from build123d import *

# Parameters (mm, degrees)
F1_DEPTH = 30
F3_DEPTH = 4.4
F4_DEPTH = 2
F5_DEPTH = 2.4
F7_DEPTH = 4.4


with BuildPart() as f1:
    # F0 (on Top) → F1 (new body)
    with BuildSketch(Plane.XY):
        with BuildLine():
            Line((7.8582108495, 2.1976148234), (7.8582108495, 1.5812813318))
            Line((7.8582108495, 1.5812813318), (7.8582108495, -2.1976148234))
            ThreePointArc((7.8582108495, -2.1976148234), (12.3474105352, -3.8320303136), (15.2004390117, 0))
            ThreePointArc((15.2004390117, 0), (12.3474105352, 3.8320303136), (7.8582108495, 2.1976148234))
        make_face()
        with BuildLine():
            ThreePointArc((8.9505391584, 1.5812813318), (12.0296782424, 2.6219958616), (13.9504390117, 0))
            ThreePointArc((13.9504390117, 0), (10.3711997809, -2.6219958616), (8.9505391584, 1.5812813318))
        make_face(mode=Mode.SUBTRACT)
        with BuildLine():
            Line((7.8582108495, -2.1976148234), (7.8582108495, 1.5812813318))
            Line((7.8582108495, 1.5812813318), (7.5262657237, 1.5812813318))
            ThreePointArc((7.5262657237, 1.5812813318), (7.2157826444, -0.3500194778), (7.8582108495, -2.1976148234))
        make_face()
        with BuildLine():
            Line((7.5262657237, 1.5812813318), (7.8582108495, 1.5812813318))
            Line((7.8582108495, 1.5812813318), (7.8582108495, 2.1976148234))
            ThreePointArc((7.8582108495, 2.1976148234), (7.6787293316, 1.8967237357), (7.5262657237, 1.5812813318))
        make_face()
        with BuildLine():
            ThreePointArc((7.8582108495, -2.1976148234), (7.2157826444, -0.3500194778), (7.5262657237, 1.5812813318))
            Line((7.5262657237, 1.5812813318), (-7.1725568309, 1.5812813318))
            ThreePointArc((-7.1725568309, 1.5812813318), (-6.9290335283, 0.8072505337), (-6.8467301189, 0))
            ThreePointArc((-6.8467301189, 0), (-7.0146998053, -1.1469715235), (-7.5045019567, -2.1976148234))
            Line((-7.5045019567, -2.1976148234), (7.8582108495, -2.1976148234))
        make_face()
        with BuildLine():
            Line((-7.1725568309, 1.5812813318), (7.5262657237, 1.5812813318))
            ThreePointArc((7.5262657237, 1.5812813318), (7.6787293316, 1.8967237357), (7.8582108495, 2.1976148234))
            Line((7.8582108495, 2.1976148234), (7.8582108495, 2.2023851766))
            Line((7.8582108495, 2.2023851766), (-7.5076434872, 2.2023851766))
            ThreePointArc((-7.5076434872, 2.2023851766), (-7.3263755669, 1.8992376967), (-7.1725568309, 1.5812813318))
        make_face()
        with BuildLine():
            ThreePointArc((-6.8467301189, 0), (-6.9290335283, 0.8072505337), (-7.1725568309, 1.5812813318))
            Line((-7.1725568309, 1.5812813318), (-7.5076434872, 1.5812813318))
            Line((-7.5076434872, 1.5812813318), (-7.5076434872, -2.1976148234))
            Line((-7.5076434872, -2.1976148234), (-7.5045019567, -2.1976148234))
            ThreePointArc((-7.5045019567, -2.1976148234), (-7.0146998053, -1.1469715235), (-6.8467301189, 0))
        make_face()
        with BuildLine():
            Line((-7.5076434872, 1.5812813318), (-7.1725568309, 1.5812813318))
            ThreePointArc((-7.1725568309, 1.5812813318), (-7.3263755669, 1.8992376967), (-7.5076434872, 2.2023851766))
            Line((-7.5076434872, 2.2023851766), (-7.5076434872, 1.5812813318))
        make_face()
        with BuildLine():
            ThreePointArc((-7.5076434872, 2.2023851766), (-14.8467290993, -0.0028559361), (-7.5045019567, -2.1976148234))
            Line((-7.5045019567, -2.1976148234), (-7.5076434872, -2.1976148234))
            Line((-7.5076434872, -2.1976148234), (-7.5076434872, 1.5812813318))
            Line((-7.5076434872, 1.5812813318), (-7.5076434872, 2.2023851766))
        make_face()
        with BuildLine():
            ThreePointArc((-8.0967301189, 0), (-13.4687259805, -0.8292392307), (-8.5968302656, 1.5812813318))
            ThreePointArc((-8.5968302656, 1.5812813318), (-8.2247342573, 0.8292392307), (-8.0967301189, 0))
        make_face(mode=Mode.SUBTRACT)
    extrude(amount=F1_DEPTH)

    # F2 (on face) → F3 (cut, through all)
    with BuildSketch(Plane.XZ.offset(2.1976148234)):
        with BuildLine():
            Line((3.1768544464, 18.5), (3.1768544464, 21))
            ThreePointArc((3.1768544464, 21), (0.1768544464, 23), (-2.8231455536, 21))
            Line((-2.8231455536, 21), (-2.8231455536, 18.5))
            ThreePointArc((-2.8231455536, 18.5), (0.1768544464, 16.5), (3.1768544464, 18.5))
        make_face()
    extrude(amount=-F3_DEPTH, mode=Mode.SUBTRACT)

    # F2 (on face) → F4 (cut)
    with BuildSketch(Plane.XZ.offset(2.1976148234)):
        with BuildLine():
            ThreePointArc((3.1768544464, 18.5), (3.3637416424, 19.1126225608), (3.4268544464, 19.75))
            ThreePointArc((3.4268544464, 19.75), (3.3637416424, 20.3873774392), (3.1768544464, 21))
            Line((3.1768544464, 21), (3.1768544464, 18.5))
        make_face()
        with BuildLine():
            Line((3.1768544464, 18.5), (3.1768544464, 21))
            ThreePointArc((3.1768544464, 21), (0.1768544464, 23), (-2.8231455536, 21))
            Line((-2.8231455536, 21), (-2.8231455536, 18.5))
            ThreePointArc((-2.8231455536, 18.5), (0.1768544464, 16.5), (3.1768544464, 18.5))
        make_face()
        with BuildLine():
            ThreePointArc((-2.8231455536, 21), (0.1768544464, 23), (3.1768544464, 21))
            Line((3.1768544464, 21), (3.1768544464, 27.75))
            Line((3.1768544464, 27.75), (-2.8231455536, 27.75))
            Line((-2.8231455536, 27.75), (-2.8231455536, 21))
        make_face()
        with BuildLine():
            Line((3.1768544464, 11.75), (3.1768544464, 18.5))
            ThreePointArc((3.1768544464, 18.5), (0.1768544464, 16.5), (-2.8231455536, 18.5))
            Line((-2.8231455536, 18.5), (-2.8231455536, 11.75))
            Line((-2.8231455536, 11.75), (3.1768544464, 11.75))
        make_face()
        with BuildLine():
            Line((-2.8231455536, 18.5), (-2.8231455536, 21))
            ThreePointArc((-2.8231455536, 21), (-3.0731455536, 19.75), (-2.8231455536, 18.5))
        make_face()
    extrude(amount=-F4_DEPTH, mode=Mode.SUBTRACT)

    # F5 (cut, through all): faces of the model
    f5_faces = [f1.faces().sort_by_distance(p)[0] for p in [
        (-2.9234827298, -0.1976148234, 19.75),
        (3.2771916226, -0.1976148234, 19.75),
    ]]
    extrude(f5_faces, amount=-F5_DEPTH, mode=Mode.SUBTRACT)

    # F6 (on face) → F7 (cut, through all)
    with BuildSketch(Plane.XZ.offset(2.1976148234)):
        with BuildLine():
            Line((-7.5045019567, 0), (7.8582108495, 0))
            Line((7.8582108495, 0), (7.8582108495, 2.0067730067))
            ThreePointArc((7.8582108495, 2.0067730067), (0.1768544464, 8.75), (-7.5045019567, 2.0067730067))
            Line((-7.5045019567, 2.0067730067), (-7.5045019567, 0))
        make_face()
    extrude(amount=-F7_DEPTH, mode=Mode.SUBTRACT)


solid = f1.part
Can you work these out from the model? Positions are in its coordinate system, mm. A direction names the side the tool comes from. Round coordinates to 2 decimals unless told otherwise and drop trailing zeros. Loops run counter-clockwise (first coordinate to the right, second up) from the corner with the lowest first, then second, coordinate; pieces in that order, holes last. Notation, with made-up numbers: (-11, 45.25) - (13, 45.25) arc R31 cw to (13, 70.25) - close; hole circle Ø3 at (49.25, 3). An arc over 180 degrees is marked (long way). Answer in a Markdown table with one row per item. Add a question column.
Q1. I want a section at C-C on y = -1.25. List the corners of the cut face in (x, z) for me, and give its area (3 significant figures).
Q2. For pin 1 Ø4.5 at (x, y) = (-10.85, 0) entering from +Z; pin 2 Ø0.6 at (y, z) = (1, 1) entering from -X (3 decimals); pin 3 Ø2 at (x, z) = (-1, 16.5) entering from -Y; pin 4 Ø1.6 at (x, y) = (0, -1) entering from -Z, each with a flat end and sliding along its axis, tell me the tip position at first contact or that it passes through.
Q3. We'd pull the mould along X, two halves only. Please class faces 1 (the flat face through (0, -0.198, 25)), 2 (the flat face through (0, 0, 30)): pulls with the +X half, pulls with the -X half, needs draft (parallel to the pull), parting line crosses it, or undercut.
Q4. Which directions (+Z, -Z, +X, -X, +Y, -Y) give clear straight access to the entire face, cutting with the end or side of a thin tool? Please do faces 3 (the flat face through (4, 2.202, 18)), 4 (the flat face through (0, -1, 11.75)), 5 (the flat face through (3.5, -2.198, 18.9)).
Q5. I want a section at A-A on z = 19.75. Count the separate pieces of the cut face and the enclosed holes in it, and give its area (3 significant figures).
Q6. I need wall thicknesses on L1, parallel to Z at x = 0, y = 1.25; L2, parallel to X at y = -1.2, z = 19.75; L3, parallel to X at y = -1.25, z = 18.75. Which ranges of each line are inside material? Lowest first, please.
Q7. I want a section at B-B on x = 13.5. List the corners of the cut face in (y, z) for me, and give its area (3 significant figures).
A:
| question | item | result |
|---|---|---|
| 1 | outline | (-14.65, 0) - (-13.3, 0) - (-13.3, 30) - (-14.65, 30) - close; (-8.4, 0) - (-7.5, 0) - (-7.5, 2.01) arc R7.75 cw to (7.86, 2.01) - (7.86, 0) - (8.75, 0) - (8.75, 30) - (-8.4, 30) - close; (13.65, 0) - (15, 0) - (15, 30) - (13.65, 30) - close; hole (-2.82, 11.75) - (3.18, 11.75) - (3.18, 18.5) arc R3.25 ccw to (3.18, 21) - (3.18, 27.75) - (-2.82, 27.75) - (-2.82, 21) arc R3.25 ccw to (-2.82, 18.5) - close |
| 1 | area | 389 mm^2 |
| 2 | pin 1 | through |
| 2 | pin 2 | x = -14.785 |
| 2 | pin 3 | y = -0.2 |
| 2 | pin 4 | z = 8.69 |
| 3 | face 1 | undercut |
| 3 | face 2 | needs draft |
| 4 | face 3 | +Z, -Z, +Y |
| 4 | face 4 | -Y |
| 4 | face 5 | +Z, -Z, -Y |
| 5 | separate pieces | 2 |
| 5 | enclosed holes | 2 |
| 5 | area | 88.1 mm^2 |
| 6 | L1 | 8.75 to 16.5, 23 to 30 |
| 6 | L2 | -14.66 to -13.32, -8.37 to -3.07, 3.43 to 8.73, 13.67 to 15.02 |
| 6 | L3 | -14.65 to -13.3, -8.4 to -2.92, 3.27 to 8.75, 13.65 to 15 |
| 7 | outline | (-3.27, 0) - (-1.51, 0) - (-1.51, 30) - (-3.27, 30) - close; (1.51, 0) - (3.27, 0) - (3.27, 30) - (1.51, 30) - close |
| 7 | area | 106 mm^2 |
